```python
from build123d import *

# Parameters (mm, degrees)
SKETCH1_R           = 2
BOSS_EXTRUDE1_DEPTH = 4


with BuildPart() as part:
    # Sketch1 → Boss-Extrude1 (new body)
    with BuildSketch(Plane.XY):
        Polygon((36, 20), (32, 20), (32, 10), (36, 10), (36, 0), (32, 0), (32, -10), (36, -10), (36, -20), (32, -20), (32, -30), (-32, -30), (-32, -20), (-36, -20), (-36, -10), (-32, -10), (-32, 0), (-36, 0), (-36, 10), (-32, 10), (-32, 20), (-36, 20), (-36, 30), (36, 30), align=None)
        with Locations((-7.5, 7.5)):
            Circle(SKETCH1_R, mode=Mode.SUBTRACT)
        with Locations((-7.5, -7.5)):
            Circle(SKETCH1_R, mode=Mode.SUBTRACT)
        with Locations((7.5, -7.5)):
            Circle(SKETCH1_R, mode=Mode.SUBTRACT)
        with Locations((7.5, 7.5)):
            Circle(SKETCH1_R, mode=Mode.SUBTRACT)
    extrude(amount=BOSS_EXTRUDE1_DEPTH)


solid = part.part
```
Part model, mm, in its own coordinate system. A direction names the side the tool comes from. Give positions to 0.01 mm unless a question says otherwise; leave off trailing zeros. Order: outer loops, then holes, each group sorted by start corner. A loop starts at its lowest first (then second) coordinate and runs counter-clockwise, first axis right, second up. Notation, with made-up numbers: (43.5, 58) - (82.5, 58) arc R30 ccw to (82.5, 81) - close; hole circle Ø11 at (53, 27.5). An arc over 180 degrees is marked (long way). Use one line per item in the form item = value.
Item 1: Slice it at A-A on y = 7.5. Give the cut face in (x, z).
Solution:
outline = (-36, 0) - (-9.5, 0) - (-9.5, 4) - (-36, 4) - close; (-5.5, 0) - (5.5, 0) - (5.5, 4) - (-5.5, 4) - close; (9.5, 0) - (36, 0) - (36, 4) - (9.5, 4) - close
Item 2: Which spindle directions (+Z, -Z, +X, -X, +Y, -Y) get a long thin tool onto all of the face, cutting with end or side? Do faces 4 (the face through (-34, 0, 2)), 5 (the face through (32, -5, 2)), 6 (the face through (1, 0, 0)). Say none if no direction does.
Solution:
face_4 = +Z, -Z, -X
face_5 = +Z, -Z, +X
face_6 = -Z, +X, -X, +Y, -Y
Item 3: Pin check, flat tips, straight feed: pin 1 Ø3 at (x, y) = (-7.5, -7.5) entering from -Z (3 decimals); pin 2 Ø2 at (x, z) = (-35, 2) entering from -Y; pin 3 Ø1.2 at (y, z) = (17, 2) entering from -X. Stop position of each tip, or through.
Solution:
pin_1 = through
pin_2 = -20
pin_3 = -32
Item 4: Slice it at B-B on x = -7.5. Give the cut face in (y, z).
Solution:
outline = (-30, 0) - (-9.5, 0) - (-9.5, 4) - (-30, 4) - close; (-5.5, 0) - (5.5, 0) - (5.5, 4) - (-5.5, 4) - close; (9.5, 0) - (30, 0) - (30, 4) - (9.5, 4) - close
Item 5: Slice it at C-C on z = 3. Give the cut face in (x, y).
Solution:
outline = (-36, -20) - (-32, -20) - (-32, -30) - (32, -30) - (32, -20) - (36, -20) - (36, -10) - (32, -10) - (32, 0) - (36, 0) - (36, 10) - (32, 10) - (32, 20) - (36, 20) - (36, 30) - (-36, 30) - (-36, 20) - (-32, 20) - (-32, 10) - (-36, 10) - (-36, 0) - (-32, 0) - (-32, -10) - (-36, -10) - close; hole circle Ø4 at (-7.5, -7.5); hole circle Ø4 at (-7.5, 7.5); hole circle Ø4 at (7.5, -7.5); hole circle Ø4 at (7.5, 7.5)
Item 6: Two-plate mould, pull along Y, no slides. Class faces 1 (the face through (34, -20, 2)), 2 (the face through (-34, 20, 2)), 3 (the face through (36, 25, 2)): released by +Y, released by -Y, zero draft, split by the parting line, or undercut.
Solution:
face_1 = released by -Y
face_2 = undercut
face_3 = zero draft
Item 7: Probe probe 1 along Y at (x, z) = (-7.5, 1.6); probe 2 along X at (y, z) = (7, 0.45); probe 3 along X at (y, z) = (13, 0.55). List the from-to ranges inside material, lowest first. Write a range as from..to.
Solution:
probe_1 = -30..-9.5, -5.5..5.5, 9.5..30
probe_2 = -36..-9.44, -5.56..5.56, 9.44..36
probe_3 = -32..32
